Source: three-view drawing plus pictorial views. Frame: mm from the lowest corner of the part. A direction names the side the tool comes from. Round coordinates to 2 decimals unless told otherwise and drop trailing zeros. Write each loop counter-clockwise with the first axis right and the second up, starting at its lowest first coordinate (ties: lowest second). Pieces come first, ordered by that corner, then holes. Notation, with made-up numbers: M -19,-30 L -7,-30 A14 cw -7,-16 Z; hole C 81.25,83.25 d11. An arc over 180 degrees is marked long. Answer in a Markdown table with one row per item.
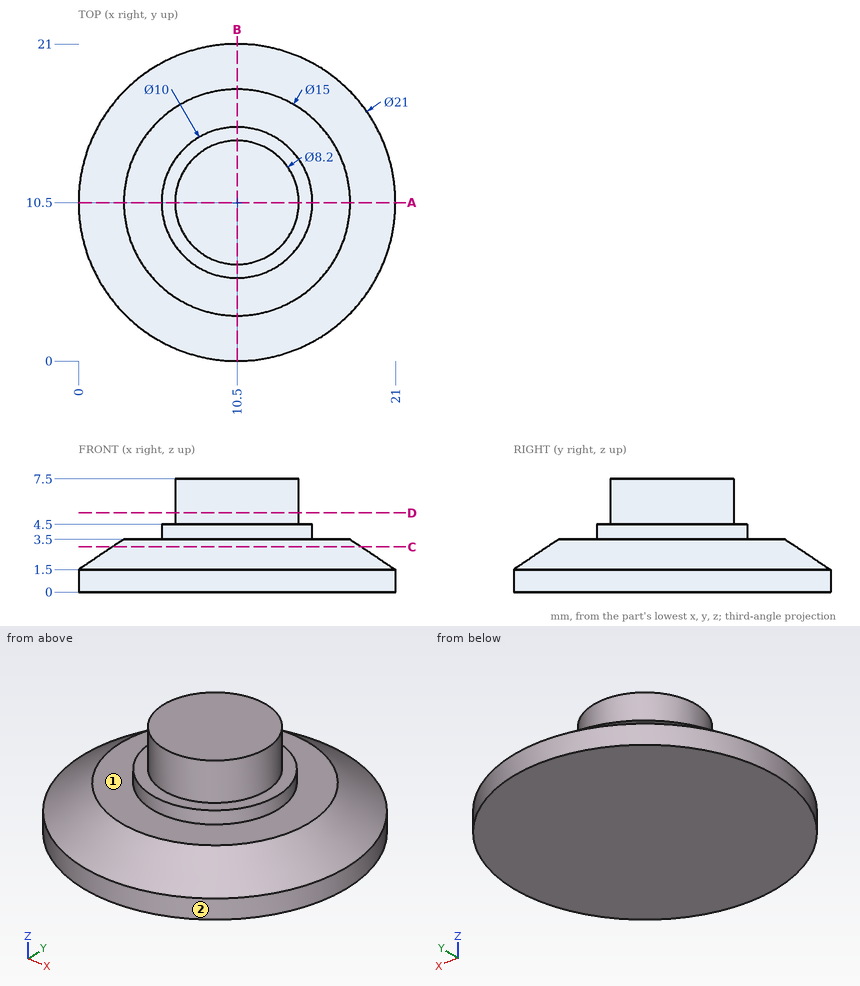
Q1. Section C-C (z = 3). Return loops of the section in (x, y), and give its area (3 significant figures).
Solutions:
| item | result |
|---|---|
| outline | C 10.5,10.5 d16.5 |
| area | 214 mm2 |
Q2. Section A-A (y = 10.5). Return loops of the section in (x, z).
Solutions:
| item | result |
|---|---|
| outline | M 0,0 L 21,0 L 21,1.5 L 18,3.5 L 15.5,3.5 L 15.5,4.5 L 14.6,4.5 L 14.6,7.5 L 6.4,7.5 L 6.4,4.5 L 5.5,4.5 L 5.5,3.5 L 3,3.5 L 0,1.5 Z |
Q3. Access query for the marked faces 1 and 2. Directions: +Z, -Z, +X, -X, +Y, -Y. A direction counts if a zero-diameter tool reaches every point of the face in a straight line with its end or side. Return the directions, or none.
Solutions:
| item | result |
|---|---|
| face 1 | +Z |
| face 2 | +Z, -Z |
Q4. Material intervals for probe 1 along Z at (x, y) = (14, 5.75); probe 2 along X at (y, z) = (7, 2.25); probe 3 along Z at (x, y) = (18.5, 17), sorted ascending.
Solutions:
| item | result |
|---|---|
| probe 1 | z = 0 to 3.5 |
| probe 2 | x = 1.8 to 19.2 |
| probe 3 | z = 0 to 1.63 |
Q5. Contact query for flat-ended pins moving along their axis: pin 1 Ø4 at (x, y) = (11, 2) entering from +Z; pin 2 Ø3 at (x, z) = (3, 3.5) entering from -Y; pin 3 Ø4 at (y, z) = (5.5, 2) entering from +X. Output: stop coordinate, or through.
Solutions:
| item | result |
|---|---|
| pin 1 | stops at z = 3.5 |
| pin 2 | stops at y = 3.88 |
| pin 3 | stops at x = 20.54 |
Q6. Section D-D (z = 5.25). Return loops of the section in (x, y), and give its area (3 significant figures).
Solutions:
| item | result |
|---|---|
| outline | C 10.5,10.5 d8.2 |
| area | 52.8 mm2 |
